```python
from build123d import *

# Parameters (mm, degrees)
EXTRUDE_1_DEPTH     = 10
SKETCH_3_W          = 4
SKETCH_3_H          = 24
EXTRUDE_2_DEPTH     = 120
CUT_EXTRUDE_1_DEPTH = 120


with BuildPart() as part:
    # 草图2 → 凸台-拉伸1 (new body)
    with BuildSketch(Plane.XY):
        with BuildLine():
            Line((-46, 0), (-42, 0))
            ThreePointArc((-42, 0), (0, 42), (42, 0))
            Line((42, 0), (46, 0))
            ThreePointArc((46, 0), (0, 46), (-46, 0))
        make_face()
    extrude(amount=EXTRUDE_1_DEPTH)

    # 草图3 → 凸台-拉伸2 (add)
    with BuildSketch(Plane(origin=(0, 0, 0), x_dir=(-1, 0, 0), z_dir=(0, 0, -1))):
        with Locations((-44, 0)):
            Rectangle(SKETCH_3_W, SKETCH_3_H)
        with Locations((44, 0)):
            Rectangle(SKETCH_3_W, SKETCH_3_H)
    extrude(amount=-EXTRUDE_2_DEPTH)

    # 草图4 → 切除-拉伸1 (cut)
    with BuildSketch(Plane.ZY.offset(46)):
        with BuildLine():
            Line((114, 0), (114, -12))
            Line((114, -12), (126, -12))
            ThreePointArc((126, -12), (134.485281374, 8.485281374), (114, 0))
        make_face()
    extrude(amount=-CUT_EXTRUDE_1_DEPTH, mode=Mode.SUBTRACT)


solid = part.part
```
Work out the finished part from the listing and answer in its coordinate system (mm). A direction names the side the tool comes from. Round coordinates to 2 decimals unless told otherwise and drop trailing zeros. Loops run counter-clockwise (first coordinate to the right, second up) from the corner with the lowest first, then second, coordinate; pieces in that order, holes last. Notation, with made-up numbers: (-21.75, 52.25) -> (-14.75, 52.25) arc R23 ccw to (-14.75, 89.25) -> close; hole circle Ø7 at (58.5, -38.75). An arc over 180 degrees is marked (long way). Write each question's results on one line, items separated by ' | '. Start each with the question number.
1. Given pin 1 Ø1.2 at (x, y) = (-44.5, -8.5) entering from +Z; pin 2 Ø1.2 at (x, z) = (44.5, 81.5) entering from +Y; pin 3 Ø23 at (x, y) = (-21.5, 31.5) entering from +Z, each flat-ended and moving along its own axis, determine where each tip first touches the part or whether it passes through.
2. A tool of negligible diameter and unlimited length cuts with its end or side. For faces 4 (the face through (44, -6, 114)), 5 (the face through (0.842, 45.992, 4.93)), from which of +Z, -Z, +X, -X, +Y, -Y can it reach the whole face along a straight path? Write none if from no direction.
3. Section A-A (z = 93.5) is taken. Determine the outline of the cut face in (x, y).
4. Section B-B (y = -6) is taken. Determine the outline of the cut face in (x, z).
5. Find the intervals of material crossed by probe 1 along X at (y, z) = (6.5, 89); probe 2 along Z at (x, y) = (-35.5, 28), in increasing order. Write a range as from..to.
6. Section D-D (x = 12.5) is taken. Determine the outline of the cut face in (y, z), plus the area to 3 significant figures.
7. For a pull along X with two mould halves and no side action, classify faces 1 (the face through (43.972, 6.076, 115.652)), 2 (the face through (-0.92, 41.99, 4.93)), 3 (the face through (46, 0, 59)) as +X half, -X half, draft (parallel to the pull), parting line (faces both ways), or undercut.
8. Section C-C (y = 3.5) is taken. Determine the outline of the cut face in (x, z), plus the area to 3 significant figures.
Evaluation:
1) pin 1: stops at z = 114 | pin 2: stops at y = 12 | pin 3: stops at z = 10
2) face 4: +Z, +X, -X, -Y | face 5: +Z, -Z, +Y
3) outline: (-46, -12) -> (-42, -12) -> (-42, 12) -> (-46, 12) -> close; (42, -12) -> (46, -12) -> (46, 12) -> (42, 12) -> close
4) outline: (-46, 0) -> (-42, 0) -> (-42, 114) -> (-46, 114) -> close; (42, 0) -> (46, 0) -> (46, 114) -> (42, 114) -> close
5) probe 1: x = -46..-42, 42..46 | probe 2: z = 0..10
6) outline: (40.1, 0) -> (44.27, 0) -> (44.27, 10) -> (40.1, 10) -> close | area: 41.7 mm2
7) face 1: draft | face 2: undercut | face 3: +X half
8) outline: (-46, 0) -> (-41.85, 0) -> (-41.85, 10) -> (-42, 10) -> (-42, 114.52) -> (-46, 114.52) -> close; (41.85, 0) -> (46, 0) -> (46, 114.52) -> (42, 114.52) -> (42, 10) -> (41.85, 10) -> close | area: 919 mm2
